Source: three-view drawing plus pictorial views. Frame: mm from the lowest corner of the part. A direction names the side the tool comes from. Coordinates: 2 decimals unless noted, no trailing zeros. Order: outer loops, then holes, each group sorted by start corner. A loop starts at its lowest first (then second) coordinate and runs counter-clockwise, first axis right, second up. Notation, with made-up numbers: (-34.5, 63) -> (16.5, 63) arc R21 ccw to (16.5, 76) -> close; hole circle Ø10 at (65, 65). An arc over 180 degrees is marked (long way). Use one line per item in the form item = value. Start each with the question number.
1) Ray query, line 1 along X through (y, z) = (1.55, 1.6); line 2 along X through (y, z) = (1.8, 0.55); line 3 along Z through (x, y) = (6, 1.8). Return the intervals inside material, ascending.
2) Draft query along Z for the marked faces 4, 5, 6 and 7. Return one class per face: pulls with the +Z half, pulls with the -Z half, needs draft (parallel to the pull), parting line crosses it, or undercut.
3) Section query C-C on y = 0.4. Output: boundary loops of the cut face in (x, z).
4) Section query A-A on z = 0.7. Output: boundary loops of the cut face in (x, y), then the cut area to 3 significant figures.
5) Section query B-B on x = 5.5. Output: boundary loops of the cut face in (y, z).
6) Access query for the marked faces 1, 2 and 3. Directions: +Z, -Z, +X, -X, +Y, -Y. A direction counts if a zero-diameter tool reaches every point of the face in a straight line with its end or side. Return the directions, or none.
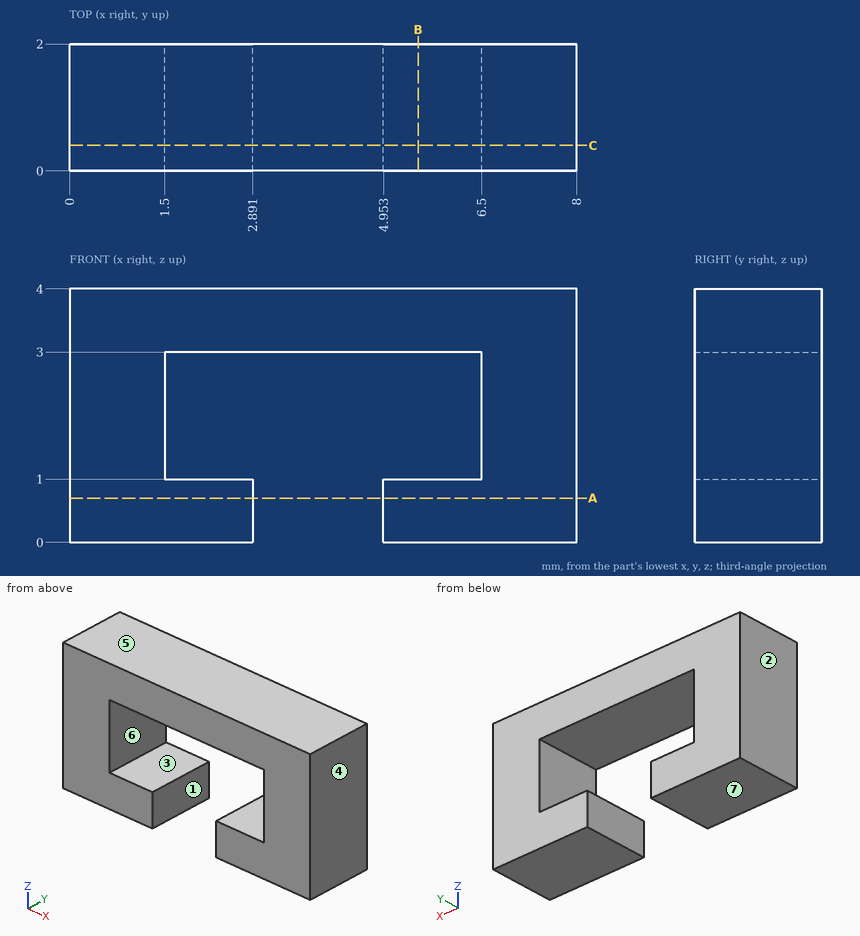
Answers below:
q1.line_1 = 0 to 1.5, 6.5 to 8
q1.line_2 = 0 to 2.89, 4.95 to 8
q1.line_3 = 0 to 1, 3 to 4
q2.face_4 = needs draft
q2.face_5 = pulls with the +Z half
q2.face_6 = undercut
q2.face_7 = pulls with the -Z half
q3.outline = (0, 0) -> (2.89, 0) -> (2.89, 1) -> (1.5, 1) -> (1.5, 3) -> (6.5, 3) -> (6.5, 1) -> (4.95, 1) -> (4.95, 0) -> (8, 0) -> (8, 4) -> (0, 4) -> close
q4.outline = (0, 0) -> (2.89, 0) -> (2.89, 2) -> (0, 2) -> close; (4.95, 0) -> (8, 0) -> (8, 2) -> (4.95, 2) -> close
q4.area = 11.9 mm^2
q5.outline = (0, 0) -> (2, 0) -> (2, 1) -> (0, 1) -> close; (0, 3) -> (2, 3) -> (2, 4) -> (0, 4) -> close
q6.face_1 = -Z, +Y, -Y
q6.face_2 = +Z, -Z, -X, +Y, -Y
q6.face_3 = +Y, -Y
